For this review, take the finished solid that the model builds, in its own axes (mm). Coordinates: 2 decimals unless noted, no trailing zeros. Write each loop counter-clockwise with the first axis right and the second up, starting at its lowest first coordinate (ties: lowest second). Pieces come first, ordered by that corner, then holes. Notation, with made-up numbers: M -7,81 L 52,81 A29 ccw 52,119 Z; hole C 26,59 d5. An arc over 180 degrees is marked long. One line per question, with ' | ' between items.
from build123d import *

# Parameters (mm, degrees)
F1_DEPTH = 0.381
F2_R     = 3.175
F3_DEPTH = 7.62
F4_R     = 1.905
F5_DEPTH = 7.62


with BuildPart() as f1:
    # F0 (on Front) → F1 (new body, symmetric)
    with BuildSketch(Plane.XZ):
        with BuildLine():
            Line((0, 16.9071391262), (0, 0))
            ThreePointArc((0, 0), (4.3273821072, 2.7700813861), (3.623545871, 7.8596983992))
            ThreePointArc((3.623545871, 7.8596983992), (2.2605059715, 11.8351901014), (3.9847012446, 15.6678866329))
            ThreePointArc((3.9847012446, 15.6678866329), (5.5496385017, 18.3998177093), (5.4302954357, 21.5459634876))
            Line((5.4302954357, 21.5459634876), (0, 38.1))
            Line((0, 38.1), (0, 22.6221391262))
            ThreePointArc((0, 22.6221391262), (2.0205576272, 21.7851967534), (2.8575, 19.7646391262))
            ThreePointArc((2.8575, 19.7646391262), (2.0205576272, 17.744081499), (0, 16.9071391262))
        make_face()
        with BuildLine():
            ThreePointArc((-3.623545871, 7.8596983992), (-4.3273821072, 2.7700813861), (0, 0))
            Line((0, 0), (0, 16.9071391262))
            ThreePointArc((0, 16.9071391262), (-2.8575, 19.7646391262), (0, 22.6221391262))
            Line((0, 22.6221391262), (0, 38.1))
            Line((0, 38.1), (-5.4302954357, 21.5459634876))
            ThreePointArc((-5.4302954357, 21.5459634876), (-5.5496385017, 18.3998177093), (-3.9847012446, 15.6678866329))
            ThreePointArc((-3.9847012446, 15.6678866329), (-2.2605059715, 11.8351901014), (-3.623545871, 7.8596983992))
        make_face()
    extrude(amount=F1_DEPTH, both=True)

    # F2 (on face) → F3 (join)
    with BuildSketch(Plane(origin=(0, 0.381, 0), x_dir=(-1, 0, 0), z_dir=(0, 1, 0))):
        with Locations((0, 4.7651283676)):
            Circle(F2_R)
    extrude(amount=F3_DEPTH)

    # F4 (on face) → F5 (cut)
    with BuildSketch(Plane(origin=(0, 8.001, 0), x_dir=(-1, 0, 0), z_dir=(0, 1, 0))):
        with Locations((0, 4.7651283676)):
            Circle(F4_R)
    extrude(amount=-F5_DEPTH, mode=Mode.SUBTRACT)


solid = f1.part
1. Take a section at C-C on z = 31. State the section outline as (x, y) points.
Computed values:
outline: M -2.33,-0.38 L 2.33,-0.38 L 2.33,0.38 L -2.33,0.38 Z
2. For line 1 along Z through (x, y) = (0, 3.25); line 2 along Y through (x, z) = (-1.5, 33); line 3 along Z through (x, y) = (-1.5, 7.5), list the stretches that pass through material, from the lowest coordinate up.
Computed values:
line 1: z = 1.59 to 2.86, 6.67 to 7.94 | line 2: y = -0.38 to 0.38 | line 3: z = 1.97 to 3.59, 5.94 to 7.56
3. Draft analysis for pull direction X (two halves, no side actions). For faces 1 (the flat face through (0, 0.381, 5)), 2 (the flat face through (0, 0.381, 15)), 3 (the cylindrical face through (0.413, 4.138, 7.913)), 4 (the cylindrical face through (0.413, 4.244, 2.905)), state which applies: pulls with the +X half, pulls with the -X half, needs draft (parallel to the pull), parting line crosses it, or undercut.
Computed values:
face 1: undercut | face 2: needs draft | face 3: parting line crosses it | face 4: undercut
4. Clearance check with flat-ended pins moving along their axes: P1, Ø3, axis at x = 4, y = 2, coming from the -Z side; P2, Ø5, axis at y = 2, z = 28.5, coming from the +X side; P3, Ø1.5, axis at x = 0, z = 16.5, coming from the +Y side. State where each tip first meets the part, or that it passes through.
Computed values:
P1: stops at z = 2.81 | P2: stops at x = 3.77 | P3: stops at y = 0.38
5. Take a section at A-A on y = 2. State the section outline as (x, z) points (3 decimals), plus the area to 3 significant figures.
Computed values:
outline: C 0,4.765 d6.35; hole C 0,4.765 d3.81 | area: 20.3 mm2
6. Take a section at D-D on x = -1.5. State the section outline as (y, z) points, plus the area to 3 significant figures.
Computed values:
outline: M -0.38,0.24 L 0.38,0.24 L 0.38,1.97 L 8,1.97 L 8,3.59 L 0.38,3.59 L 0.38,5.94 L 8,5.94 L 8,7.56 L 0.38,7.56 L 0.38,17.33 L -0.38,17.33 Z; M -0.38,22.2 L 0.38,22.2 L 0.38,33.53 L -0.38,33.53 Z | area: 46.4 mm2
7. Take a section at B-B on x = 1. State the section outline as (y, z) points, plus the area to 3 significant figures.
Computed values:
outline: M -0.38,0.11 L 0.38,0.11 L 0.38,1.75 L 8,1.75 L 8,3.14 L 0.38,3.14 L 0.38,6.39 L 8,6.39 L 8,7.78 L 0.38,7.78 L 0.38,17.09 L -0.38,17.09 Z; M -0.38,22.44 L 0.38,22.44 L 0.38,35.05 L -0.38,35.05 Z | area: 43.8 mm2
